Drawing for the job (mm, zero at the part's lowest x, y, z). Coordinates: 2 decimals unless noted, no trailing zeros. Write each loop counter-clockwise with the first axis right and the second up, starting at its lowest first coordinate (ties: lowest second). Pieces come first, ordered by that corner, then holes.
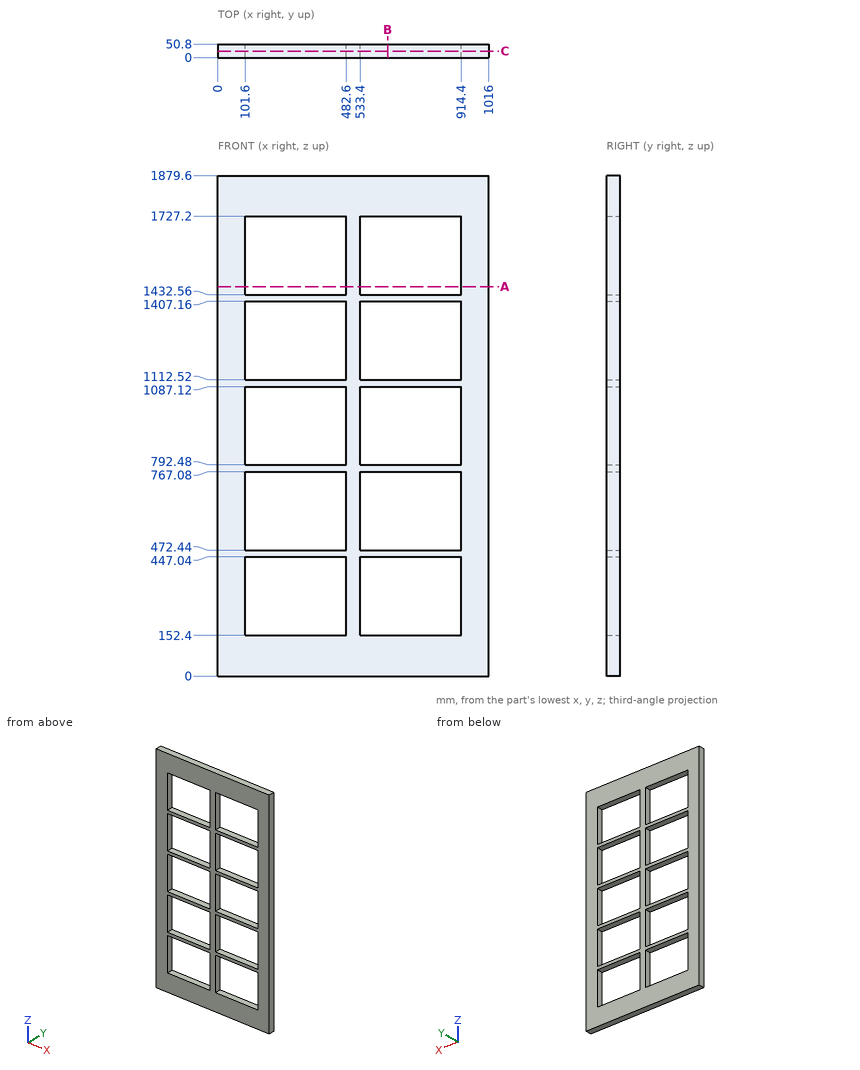
Item 1: Saw through at A-A, the plane z = 1462. Write the cut outline in (x, y).
Item 2: Flat gauge pin, fed straight in: pin 1 Ø8 at (x, y) = (643, 44) entering from -Z. Where does the tip first touch, or does it go through?
Item 3: Saw through at B-B, the plane x = 637. Write the cut outline in (y, z).
Item 4: Wall check: line 1 along X through (y, z) = (45, 219); line 2 along Z through (x, y) = (656.5, 30). Give the ranges that are in metal, low to high.
Item 5: Saw through at C-C, the plane y = 24.5. State how many separate pieces and enclosed holes the cut face has, and give its area (3 significant figures).
Working result:
1. outline: (0, 0) - (101.6, 0) - (101.6, 50.8) - (0, 50.8) - close; (482.6, 0) - (533.4, 0) - (533.4, 50.8) - (482.6, 50.8) - close; (914.4, 0) - (1016, 0) - (1016, 50.8) - (914.4, 50.8) - close
2. pin 1: stops at z = 0
3. outline: (0, 0) - (50.8, 0) - (50.8, 152.4) - (0, 152.4) - close; (0, 447.04) - (50.8, 447.04) - (50.8, 472.44) - (0, 472.44) - close; (0, 767.08) - (50.8, 767.08) - (50.8, 792.48) - (0, 792.48) - close; (0, 1087.12) - (50.8, 1087.12) - (50.8, 1112.52) - (0, 1112.52) - close; (0, 1407.16) - (50.8, 1407.16) - (50.8, 1432.56) - (0, 1432.56) - close; (0, 1727.2) - (50.8, 1727.2) - (50.8, 1879.6) - (0, 1879.6) - close
4. line 1: x = 0 to 101.6, 482.6 to 533.4, 914.4 to 1016
4. line 2: z = 0 to 152.4, 447.04 to 472.44, 767.08 to 792.48, 1087.12 to 1112.52, 1407.16 to 1432.56, 1727.2 to 1879.6
5. separate pieces: 1
5. enclosed holes: 10
5. area: 787,000 mm2
